from build123d import *

# Parameters (mm, degrees)
SKETCH1_R      = 123.825
EXTRUDE1_DEPTH = 76.2
SKETCH4_W      = 17.455227324
SKETCH4_H      = 66.2
EXTRUDE7_DEPTH = 191.975656171
SKETCH8_R      = 103.876598788
EXTRUDE8_DEPTH = 61.357082


with BuildPart() as part:
    # Sketch1 → Extrude1 (new body)
    with BuildSketch(Plane.XY):
        with Locations(Location((0, 0, 0), (0, 0, 180))):
            Circle(SKETCH1_R)
    extrude(amount=EXTRUDE1_DEPTH)

    # Sketch4 → Cut-Revolve1 (revolve, cut)
    with BuildSketch(Plane(origin=(0, 0, 0), x_dir=(1, 0, 0), z_dir=(0, 1, 0)), mode=Mode.PRIVATE) as cut_revolve1_sk:
        with Locations((115.097386338, -38.1)):
            Rectangle(SKETCH4_W, SKETCH4_H)
    revolve(cut_revolve1_sk.sketch.rotate(Axis((0, 0, 0), (0, 0, 1)), 180), axis=Axis((0, 0, 0), (0, 0, 1)), mode=Mode.SUBTRACT)

    # Sketch2 → Extrude7 (cut, through all)
    with BuildSketch(Plane(origin=(0, 0, 0), x_dir=(-1, 0, 0), z_dir=(0, 0, -1))):
        with BuildLine():
            add(Edge.make_bspline(
                [(-87.364978695, -16.449027254), (-61.27965147, -10.813441939), (-48.861717362, -2.569537789)],
                knots=[0, 0, 0, 0.288609818, 0.288609818, 0.288609818], degree=2))
            Line((-48.861717362, -2.569537789), (-55.5625, 18.053350622))
            Line((-55.5625, 18.053350622), (-42.187847239, 27.77060465))
            add(Edge.make_bspline(
                [(-42.187847239, 27.77060465), (-49.93088885, 39.603142144), (-70.682590657, 53.918284265)],
                knots=[0.718431192, 0.718431192, 0.718431192, 1, 1, 1], degree=2))
            Line((-70.682590657, 53.918284265), (-86.502301571, 20.507604026))
            Line((-86.502301571, 20.507604026), (-87.364978695, -16.449027254))
        make_face()
        with BuildLine():
            Line((-86.502301571, 20.507604026), (-70.682590657, 53.918284265))
            ThreePointArc((-70.682590657, 53.918284265), (-80.348248112, 38.044303454), (-86.502301571, 20.507604026))
        make_face()
        with BuildLine():
            ThreePointArc((-86.502301571, 20.507604026), (-88.875789367, 2.074623896), (-87.364978695, -16.449027254))
            Line((-87.364978695, -16.449027254), (-86.502301571, 20.507604026))
        make_face()
        with BuildLine():
            add(Edge.make_bspline(
                [(-48.861717362, -2.569537789), (-38.943167303, 4.015098212), (-37.743952233, 12.263753494)],
                knots=[0.288609818, 0.288609818, 0.288609818, 0.519130523, 0.519130523, 0.519130523], degree=2))
            add(Edge.make_bspline(
                [(-37.743952233, 12.263753494), (-36.707150073, 19.395271291), (-42.187847239, 27.77060465)],
                knots=[0.519130523, 0.519130523, 0.519130523, 0.718431192, 0.718431192, 0.718431192], degree=2))
            Line((-42.187847239, 27.77060465), (-55.5625, 18.053350622))
            Line((-55.5625, 18.053350622), (-48.861717362, -2.569537789))
        make_face()
        with BuildLine():
            add(Edge.make_bspline(
                [(-11.353308573, -88.172061246), (-8.652259294, -61.621949174), (-12.655325381, -47.264285539)],
                knots=[0, 0, 0, 0.288609818, 0.288609818, 0.288609818], degree=2))
            Line((-12.655325381, -47.264285539), (-34.3395135, -47.264285539))
            Line((-34.3395135, -47.264285539), (-39.448176267, -31.541438244))
            add(Edge.make_bspline(
                [(-39.448176267, -31.541438244), (-53.094319601, -35.249053252), (-73.121457317, -50.561472287)],
                knots=[0.718431192, 0.718431192, 0.718431192, 1, 1, 1], degree=2))
            Line((-73.121457317, -50.561472287), (-46.234571681, -75.931379426))
            Line((-46.234571681, -75.931379426), (-11.353308573, -88.172061246))
        make_face()
        with BuildLine():
            add(Edge.make_bspline(
                [(-12.655325381, -47.264285539), (-15.852685829, -35.796419447), (-23.32704535, -32.106923477)],
                knots=[0.288609818, 0.288609818, 0.288609818, 0.519130523, 0.519130523, 0.519130523], degree=2))
            add(Edge.make_bspline(
                [(-23.32704535, -32.106923477), (-29.789132335, -28.917105832), (-39.448176267, -31.541438244)],
                knots=[0.519130523, 0.519130523, 0.519130523, 0.718431192, 0.718431192, 0.718431192], degree=2))
            Line((-39.448176267, -31.541438244), (-34.3395135, -47.264285539))
            Line((-34.3395135, -47.264285539), (-12.655325381, -47.264285539))
        make_face()
        with BuildLine():
            Line((-46.234571681, -75.931379426), (-73.121457317, -50.561472287))
            ThreePointArc((-73.121457317, -50.561472287), (-61.011256843, -64.659388633), (-46.234571681, -75.931379426))
        make_face()
        with BuildLine():
            ThreePointArc((-46.234571681, -75.931379426), (-29.437213878, -83.884804578), (-11.353308573, -88.172061246))
            Line((-11.353308573, -88.172061246), (-46.234571681, -75.931379426))
        make_face()
        with BuildLine():
            ThreePointArc((57.927764817, -67.435777324), (70.682590657, -53.918284265), (80.348248112, -38.044303454))
            Line((80.348248112, -38.044303454), (57.927764817, -67.435777324))
        make_face()
        with BuildLine():
            add(Edge.make_bspline(
                [(80.348248112, -38.044303454), (55.932261147, -27.271017104), (41.040296138, -26.641397128)],
                knots=[0, 0, 0, 0.288609818, 0.288609818, 0.288609818], degree=2))
            Line((41.040296138, -26.641397128), (34.3395135, -47.264285539))
            Line((34.3395135, -47.264285539), (17.807533512, -47.264285539))
            add(Edge.make_bspline(
                [(17.807533512, -47.264285539), (17.116794728, -61.388255125), (25.491044728, -85.16699266)],
                knots=[0.718431192, 0.718431192, 0.718431192, 1, 1, 1], degree=2))
            Line((25.491044728, -85.16699266), (57.927764817, -67.435777324))
            Line((57.927764817, -67.435777324), (80.348248112, -38.044303454))
        make_face()
        with BuildLine():
            add(Edge.make_bspline(
                [(41.040296138, -26.641397128), (29.145668647, -26.138502105), (23.32704535, -32.106923477)],
                knots=[0.288609818, 0.288609818, 0.288609818, 0.519130523, 0.519130523, 0.519130523], degree=2))
            add(Edge.make_bspline(
                [(23.32704535, -32.106923477), (18.296453795, -37.267025552), (17.807533512, -47.264285539)],
                knots=[0.519130523, 0.519130523, 0.519130523, 0.718431192, 0.718431192, 0.718431192], degree=2))
            Line((17.807533512, -47.264285539), (34.3395135, -47.264285539))
            Line((34.3395135, -47.264285539), (41.040296138, -26.641397128))
        make_face()
        with BuildLine():
            Line((57.927764817, -67.435777324), (25.491044728, -85.16699266))
            ThreePointArc((25.491044728, -85.16699266), (42.641217687, -78.006003322), (57.927764817, -67.435777324))
        make_face()
        with BuildLine():
            add(Edge.make_bspline(
                [(61.011256843, 64.659388633), (43.220297751, 44.767533696), (38.019623302, 30.798996606)],
                knots=[0, 0, 0, 0.288609818, 0.288609818, 0.288609818], degree=2))
            Line((38.019623302, 30.798996606), (55.5625, 18.053350622))
            Line((55.5625, 18.053350622), (50.453837233, 2.330503327))
            add(Edge.make_bspline(
                [(50.453837233, 2.330503327), (63.673080521, -2.690974925), (88.875789367, -2.074623896)],
                knots=[0.718431192, 0.718431192, 0.718431192, 1, 1, 1], degree=2))
            Line((88.875789367, -2.074623896), (82.03589923, 34.253776982))
            Line((82.03589923, 34.253776982), (61.011256843, 64.659388633))
        make_face()
        with BuildLine():
            add(Edge.make_bspline(
                [(38.019623302, 30.798996606), (33.865699678, 19.641936731), (37.743952233, 12.263753494)],
                knots=[0.288609818, 0.288609818, 0.288609818, 0.519130523, 0.519130523, 0.519130523], degree=2))
            add(Edge.make_bspline(
                [(37.743952233, 12.263753494), (41.096962653, 5.884817381), (50.453837233, 2.330503327)],
                knots=[0.519130523, 0.519130523, 0.519130523, 0.718431192, 0.718431192, 0.718431192], degree=2))
            Line((50.453837233, 2.330503327), (55.5625, 18.053350622))
            Line((55.5625, 18.053350622), (38.019623302, 30.798996606))
        make_face()
        with BuildLine():
            ThreePointArc((82.03589923, 34.253776982), (73.121457317, 50.561472287), (61.011256843, 64.659388633))
            Line((61.011256843, 64.659388633), (82.03589923, 34.253776982))
        make_face()
        with BuildLine():
            Line((82.03589923, 34.253776982), (88.875789367, -2.074623896))
            ThreePointArc((88.875789367, -2.074623896), (88.893947136, -1.037382579), (88.9, 0))
            ThreePointArc((88.9, 0), (87.167085077, 17.467377571), (82.03589923, 34.253776982))
        make_face()
        with BuildLine():
            add(Edge.make_bspline(
                [(-42.641217687, 78.006003322), (-29.220648133, 54.938874521), (-17.542876698, 45.67622385)],
                knots=[0, 0, 0, 0.288609818, 0.288609818, 0.288609818], degree=2))
            Line((-17.542876698, 45.67622385), (0, 58.421869834))
            Line((0, 58.421869834), (13.374652761, 48.704615806))
            add(Edge.make_bspline(
                [(13.374652761, 48.704615806), (22.235333203, 59.725141159), (29.437213878, 83.884804578)],
                knots=[0.718431192, 0.718431192, 0.718431192, 1, 1, 1], degree=2))
            Line((29.437213878, 83.884804578), (-7.226790795, 88.605775742))
            Line((-7.226790795, 88.605775742), (-42.641217687, 78.006003322))
        make_face()
        with BuildLine():
            ThreePointArc((-7.226790795, 88.605775742), (-25.491044728, 85.16699266), (-42.641217687, 78.006003322))
            Line((-42.641217687, 78.006003322), (-7.226790795, 88.605775742))
        make_face()
        with BuildLine():
            add(Edge.make_bspline(
                [(-17.542876698, 45.67622385), (-8.215515194, 38.27788661), (0, 39.686339966)],
                knots=[0.288609818, 0.288609818, 0.288609818, 0.519130523, 0.519130523, 0.519130523], degree=2))
            add(Edge.make_bspline(
                [(0, 39.686339966), (7.102865959, 40.904042711), (13.374652761, 48.704615806)],
                knots=[0.519130523, 0.519130523, 0.519130523, 0.718431192, 0.718431192, 0.718431192], degree=2))
            Line((13.374652761, 48.704615806), (0, 58.421869834))
            Line((0, 58.421869834), (-17.542876698, 45.67622385))
        make_face()
        with BuildLine():
            Line((-7.226790795, 88.605775742), (29.437213878, 83.884804578))
            ThreePointArc((29.437213878, 83.884804578), (11.353308573, 88.172061246), (-7.226790795, 88.605775742))
        make_face()
    extrude(amount=-EXTRUDE7_DEPTH, mode=Mode.SUBTRACT)

    # Sketch5 → Revolve1 (revolve)
    with BuildSketch(Plane(origin=(0, 0, 0), x_dir=(1, 0, 0), z_dir=(0, 1, 0))):
        with BuildLine():
            Line((-123.825, -71.2), (-106.369772676, -71.2))
            Line((-106.369772676, -71.2), (-106.369772676, -5))
            Line((-106.369772676, -5), (-123.825, -5))
            ThreePointArc((-123.825, -5), (-183.480240999, -38.1), (-123.825, -71.2))
        make_face()
    revolve(axis=Axis((0, 0, 0), (0, 0, 1)))

    # Sketch8 → Extrude8 (cut)
    with BuildSketch(Plane(origin=(0, 0, 0), x_dir=(-1, 0, 0), z_dir=(0, 0, -1))):
        Circle(SKETCH8_R)
    extrude(amount=-EXTRUDE8_DEPTH, mode=Mode.SUBTRACT)


solid = part.part
The model under review builds one solid part; all positions refer to its coordinate system, in mm. A direction names the side the tool comes from. Round coordinates to 2 decimals unless told otherwise and drop trailing zeros. Write each loop counter-clockwise with the first axis right and the second up, starting at its lowest first coordinate (ties: lowest second). Pieces come first, ordered by that corner, then holes. Notation, with made-up numbers: (-10.5, 56.25) - (-1.5, 56.25) arc R31 cw to (-1.5, 95.25) - close; hole circle Ø5 at (0.25, 85). An arc over 180 degrees is marked (long way). One line per item, written item: value. Start each with the question number.
1. The part is to be moulded in two halves that separate along X. For faces 1 (the face through (28, -101, 0)), 2 (the face through (26.84, 120.88, 73.67)), say which applies: released by +X, released by -X, zero draft, split by the parting line, or undercut.
2. Consider section C-C on z = 33.5. Write out the cut boundary in (x, y).
3. To check wall thickness, follow L1, parallel to Y at x = 0, z = 37; L2, parallel to Y at x = 41.5, z = 71; L3, parallel to Z at x = -88.5, y = -78.5. State the ranges of each line that lie inside material, in increasing order. Write a range as from..to.
4. Clearance check with flat-ended pins moving along their axes: P1, Ø12, axis at y = -13.5, z = 32, coming from the -X side; P2, Ø10, axis at x = -141, z = 47, coming from the +Y side; P3, Ø6, axis at x = 114.5, z = 14.5, coming from the -Y side. State where each tip first meets the part, or that it passes through.
5. Consider section B-B on z = 52. Write out the cut boundary in (x, y).
6. Consider section A-A on y = -57. State how many separate pieces and enclosed holes the cut face has, and give its area (3 significant figures).
7. Machinability: for faces 3 (the face through (2, -2, 76.2)), 4 (the face through (22.518, -101.406, 30.249)), which of the approach directions +Z, -Z, +X, -X, +Y, -Y give a long, thin tool a straight path to every point of the face, cutting with its end or side? Answer none if there is none.
Checks:
1. face 1: undercut
1. face 2: undercut
2. outline: circle Ø366.42 at (0, 0); hole circle Ø207.75 at (0, 0)
3. L1: y = -183.46..-103.88, 103.88..183.46
3. L2: y = -160.14..-78.62, -32.15..3.94, 26.68..76.06, 78.62..160.14
3. L3: z = 0..76.2
4. P1: stops at x = -183.2
4. P2: stops at y = 121.85
4. P3: stops at y = -136.79
5. outline: circle Ø361.84 at (0, 0); hole circle Ø207.75 at (0, 0)
6. separate pieces: 3
6. enclosed holes: 0
6. area: 13,000 mm^2
7. face 3: +Z
7. face 4: -Z
